```python
from build123d import *

# Parameters (mm, degrees)
F0_W          = 55.6310900272
F0_H          = 100
F1_DEPTH      = 8
F2_W          = 2.5
F2_H          = 158.0840436167
F3_DEPTH      = 27.8165450136
F3_DEPTH_BACK = 25
F5_DEPTH      = 50


# Not quite as in the source:
# - a feature names something its author has since deleted; it is built from what else it names


with BuildPart() as f1:
    # F0 (on Front) → F1 (new body)
    with BuildSketch(Plane.XZ):
        Rectangle(F0_W, F0_H)
    extrude(amount=-F1_DEPTH)

    # F2 (on Right) → F3 (cut, two sides)
    with BuildSketch(Plane.YZ) as f3_sk:
        with Locations((3.9288233686, 7.7119854566)):
            Rectangle(F2_W, F2_H)
    extrude(amount=F3_DEPTH, mode=Mode.SUBTRACT)
    extrude(f3_sk.sketch, amount=-F3_DEPTH_BACK, mode=Mode.SUBTRACT)

    # F4 (on Top) → F5 (join, symmetric)
    with BuildSketch(Plane.XY):
        Polygon((23.6732276815, 28.1708468052), (-27.8155450136, 14.3744717422), (-27.8155450136, 8), (-23.8155450136, 8), (-23.8155450136, 11.3051637903), (24.3706528022, 24.2166165814), (23.6732276815, 20.2701286405), (27.8155450136, 20.2701286405), (27.6694063807, 28.3456489901), align=None)
    extrude(amount=F5_DEPTH, both=True)


solid = f1.part
```
Input: part model. Units: mm. Frame: model coordinates. A direction names the side the tool comes from. Round coordinates to 2 decimals unless told otherwise and drop trailing zeros. Order: outer loops, then holes, each group sorted by start corner. A loop starts at its lowest first (then second) coordinate and runs counter-clockwise, first axis right, second up. Notation, with made-up numbers: (71.25, 14) - (85.25, 14) arc R22 ccw to (85.25, 45) - close; hole circle Ø1 at (23, 85.25). An arc over 180 degrees is marked (long way). One line per question, with ' | ' between items. Start each with the question number.
1) Cut plane B-B, the plane y = 21.5. Return the cut outline in (x, z), then the cut area to 3 significant figures.
2) Pull-direction query (X, two-part tool) for faces 3 (the flat face through (-0.06, 17.67, 0.7)), 4 (the flat face through (24.027, 22.271, 0.7)), 5 (the flat face through (2, 5.179, -1)), 6 (the flat face through (-25, 4, 1)); classes: +X half, -X half, draft (parallel to the pull), parting line (faces both ways), or undercut.
3) Set-up query: faces 1 (the flat face through (27.816, 7, -1)), 2 (the flat face through (-23.816, 10, 1)). Return all of +Z, -Z, +X, -X, +Y, -Y with unobstructed straight access to the full face (end or side cutting, diameter ignored); none if empty.
4) Ray query, probe 1 along Y at (x, z) = (8.5, -14); probe 2 along Y at (x, z) = (20.5, 6.5); probe 3 along X at (y, z) = (3.5, 13). Return the intervals inside material, ascending.
5) Cut plane C-C, the plane x = 21. Return the cut outline in (y, z).
6) Cut plane D-D, the plane y = 25.75. Return the cut outline in (x, z), then the cut area to 3 significant figures.
7) Cut plane A-A, the plane z = -24.5. Return the cut outline in (x, y), then the cut area to 3 significant figures.
8) Contact query for flat-ended pins moving along their axis: P1, Ø10, axis at x = 10.5, z = -22.5, coming from the -Y side; P2, Ø1.7, axis at y = 10, z = -4.5, coming from the +X side; P3, Ø2, axis at x = -3.5, z = -37.5, coming from the +Y side; P4, Ø4, axis at x = 7, z = 0, coming from the +Y side. Output: stop coordinate, or through.
Worked out:
1) outline: (-1.22, -50) - (14.23, -50) - (14.23, 50) - (-1.22, 50) - close; (23.89, -50) - (27.79, -50) - (27.79, 50) - (23.89, 50) - close | area: 1,940 mm^2
2) face 3: undercut | face 4: undercut | face 5: draft | face 6: +X half
3) face 1: +Z, -Z, +X, +Y, -Y | face 2: +Z, -Z, +X
4) probe 1: y = 0 to 2.68, 5.18 to 8, 19.96 to 24.11 | probe 2: y = 0 to 2.68, 5.18 to 8, 23.18 to 27.32 | probe 3: x = -27.82 to -25
5) outline: (0, -50) - (2.68, -50) - (2.68, 50) - (0, 50) - close; (5.18, -50) - (8, -50) - (8, 50) - (5.18, 50) - close; (23.31, -50) - (27.45, -50) - (27.45, 50) - (23.31, 50) - close
6) outline: (14.64, -50) - (27.72, -50) - (27.72, 50) - (14.64, 50) - close | area: 1,310 mm^2
7) outline: (-27.82, 0) - (27.82, 0) - (27.82, 2.68) - (-25, 2.68) - (-25, 5.18) - (27.82, 5.18) - (27.82, 8) - (-23.82, 8) - (-23.82, 11.31) - (24.37, 24.22) - (23.67, 20.27) - (27.82, 20.27) - (27.67, 28.35) - (23.67, 28.17) - (-27.82, 14.37) - close | area: 569 mm^2
8) P1: stops at y = 0 | P2: stops at x = -23.82 | P3: stops at y = 21.16 | P4: stops at y = 24.24
